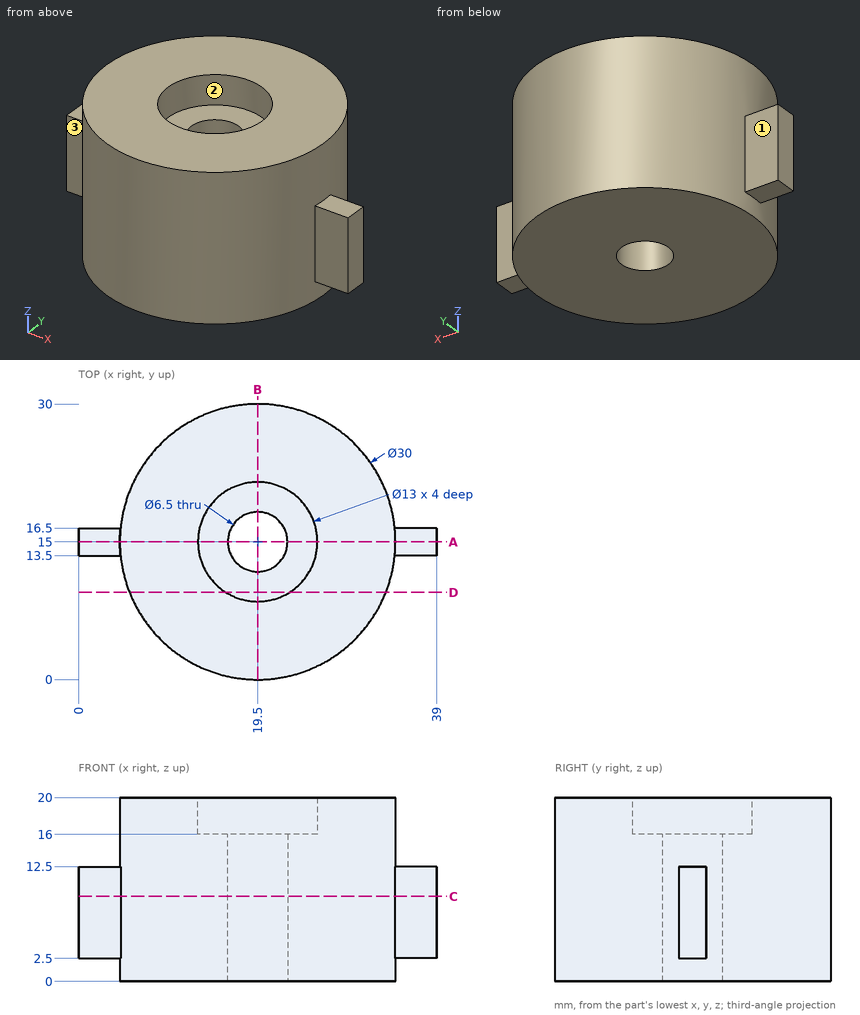
Check sheet for the drawn part. Datum: minimum x, y, z corner. Units: mm. A direction names the side the tool comes from. Coordinates: 2 decimals unless noted, no trailing zeros. Loops run counter-clockwise (first coordinate to the right, second up) from the corner with the lowest first, then second, coordinate; pieces in that order, holes last. Notation, with made-up numbers: (-27, 33) -> (4, 33) arc R22 cw to (4, 57) -> close; hole circle Ø10 at (-38.75, 50). An arc over 180 degrees is marked (long way). Answer in a Markdown table with one row per item.
1) Scan lines: line 1 along Y through (x, z) = (19.5, 3.75); line 2 along X through (y, z) = (13.25, 1.75); line 3 along Y through (x, z) = (3, 8.5). Record each from-to range of solid material in increasing order. Write a range as from..to.
The answers:
| item | result |
|---|---|
| line 1 | y = 0..11.75, 18.25..30 |
| line 2 | x = 4.6..16.76, 22.24..34.4 |
| line 3 | y = 13.5..16.5 |
2) Depth check by flat-ended pin: P1, Ø4, axis at y = 26.5, z = 12.5, coming from the -X side; P2, Ø10.5, axis at x = 22.5, y = 15.5, coming from the +Z side; P3, Ø3.5, axis at x = 1.5, y = 14.5, coming from the -Z side; P4, Ø1.4, axis at x = 36, z = 8, coming from the -Y side. Enter the tip coordinate at first touch or a pass-through.
The answers:
| item | result |
|---|---|
| P1 | stops at x = 7.89 |
| P2 | stops at z = 20 |
| P3 | stops at z = 2.5 |
| P4 | stops at y = 13.5 |
3) Section check D-D (y = 9.5). Record the cut outline in (x, z), and give its area (4 significant figures).
The answers:
| item | result |
|---|---|
| outline | (5.54, 0) -> (33.46, 0) -> (33.46, 20) -> (22.96, 20) -> (22.96, 16) -> (16.04, 16) -> (16.04, 20) -> (5.54, 20) -> close |
| area | 530.5 mm2 |
4) Section check C-C (z = 9.25). Record the cut outline in (x, y).
The answers:
| item | result |
|---|---|
| outline | (0, 13.5) -> (4.58, 13.5) arc R15 ccw to (34.42, 13.5) -> (39, 13.5) -> (39, 16.5) -> (34.42, 16.5) arc R15 ccw to (4.58, 16.5) -> (0, 16.5) -> close; hole circle Ø6.5 at (19.5, 15) |
5) Access from +Z, -Z, +X, -X, +Y, -Y to the whole of each face (thin tool, end or side, straight path). Record for the marked faces 1, 2 and 3.
The answers:
| item | result |
|---|---|
| face 1 | +Z, -Z, -X, +Y |
| face 2 | +Z |
| face 3 | +Z, -Z, -X, -Y |
6) Section check B-B (x = 19.5). Record the cut outline in (y, z), and give its area (3 significant figures).
The answers:
| item | result |
|---|---|
| outline | (0, 0) -> (11.75, 0) -> (11.75, 16) -> (8.5, 16) -> (8.5, 20) -> (0, 20) -> close; (18.25, 0) -> (30, 0) -> (30, 20) -> (21.5, 20) -> (21.5, 16) -> (18.25, 16) -> close |
| area | 444 mm2 |
7) Section check A-A (y = 15). Record the cut outline in (x, z).
The answers:
| item | result |
|---|---|
| outline | (0, 2.5) -> (4.5, 2.5) -> (4.5, 0) -> (16.25, 0) -> (16.25, 16) -> (13, 16) -> (13, 20) -> (4.5, 20) -> (4.5, 12.5) -> (0, 12.5) -> close; (22.75, 0) -> (34.5, 0) -> (34.5, 2.5) -> (39, 2.5) -> (39, 12.5) -> (34.5, 12.5) -> (34.5, 20) -> (26, 20) -> (26, 16) -> (22.75, 16) -> close |
